For this review, take the finished solid that the model builds, in its own axes (mm). A direction names the side the tool comes from. Give positions to 0.01 mm unless a question says otherwise; leave off trailing zeros. Write each loop counter-clockwise with the first axis right and the second up, starting at its lowest first coordinate (ties: lowest second). Pieces come first, ordered by that corner, then holes.
1) We need section C-C on x = -27. Give the boundary of the cut face in (y, z), and give its area (3 significant figures).
2) Wall thickness on line 1 along Y through (x, z) = (0, 4); line 2 along Y through (x, z) = (-26.5, 0.75); line 3 along X through (y, z) = (8, 2.5): over which ranges is each line inside the solid? List them lowest first.
3) We need section D-D on x = -7.5. Give the boundary of the cut face in (y, z).
4) Machinability: for faces 5 (the face through (-22, 3.687, 3)), 6 (the face through (-29, 4.738, 3)), 7 (the face through (-31.567, -4, 3)), 8 (the face through (-0.22, -21.85, 7.49)), which of the approach directions +Z, -Z, +X, -X, +Y, -Y give a long, thin tool a straight path to every point of the face, cutting with its end or side? Answer none if there is none.
5) We need section B-B on x = 0. Give the boundary of the cut face in (y, z) (3 decimals), and give its area (3 significant figures).
6) For P1, Ø1.5, axis at x = 7, y = 14.5, coming from the +Z side; P2, Ø3.5, axis at x = -25.5, z = 3, coming from the +Y side, all flat-tipped, find the tip position at first contact; note any pin that passes through.
7) Draft analysis for pull direction Z (two halves, no side actions). For faces 1 (the face through (-27.028, -4.485, 1.426)), 2 (the face through (-28.3, -5.262, 1.9)), 3 (the face through (8, -10, 7)), 4 (the face through (-27.028, 4.205, 1.426)), state which applies: pulls with the +Z half, pulls with the -Z half, needs draft (parallel to the pull), parting line crosses it, or undercut.
8) We need section A-A on z = 3.5. Give the boundary of the cut face in (x, y), and give its area (3 significant figures).
from build123d import *

# Parameters (mm, degrees)
F1_DEPTH = 7
F2_R     = 2.125
F3_DEPTH = 10
F4_R     = 1
F5_DEPTH = 1


# Not quite as in the source:
# - a feature names something its author has since deleted; it is built from what else it names


with BuildPart() as f1:
    # F0 (on Top) → F1 (new body)
    with BuildSketch(Plane.XY):
        with BuildLine():
            ThreePointArc((-23.208916684, 3.6873006871), (-23.1191027664, 4.2139159074), (-23.017341427, 4.7383534726))
            Line((-23.017341427, 4.7383534726), (-31.5671088163, 4.7383534726))
            Line((-31.5671088163, 4.7383534726), (-31.5671088163, 3.6873006871))
            Line((-31.5671088163, 3.6873006871), (-23.208916684, 3.6873006871))
        make_face()
        with BuildLine():
            Line((-31.5671088163, -5.2616465274), (-22.9033856847, -5.2616465274))
            ThreePointArc((-22.9033856847, -5.2616465274), (-23.0695849256, -4.4770806738), (-23.208916684, -3.6873006871))
            Line((-23.208916684, -3.6873006871), (-31.5671088163, -3.6873006871))
            Line((-31.5671088163, -3.6873006871), (-31.5671088163, -5.2616465274))
        make_face()
        with BuildLine():
            ThreePointArc((-22.9033856847, -5.2616465274), (2.6476816661, -23.3503700569), (23.5, 0))
            ThreePointArc((23.5, 0), (2.3814361701, 23.3790239695), (-23.017341427, 4.7383534726))
            Line((-23.017341427, 4.7383534726), (-11.5671088163, 4.7383534726))
            ThreePointArc((-11.5671088163, 4.7383534726), (2.4146573045, 12.2645599229), (12.5, 0))
            ThreePointArc((12.5, 0), (2.4146573045, -12.2645599229), (-11.5671088163, -4.7383534726))
            Line((-11.5671088163, -4.7383534726), (-11.5671088163, -5.2616465274))
            Line((-11.5671088163, -5.2616465274), (-22.9033856847, -5.2616465274))
        make_face()
        with BuildLine():
            Line((-11.5671088163, 4.7383534726), (-23.017341427, 4.7383534726))
            ThreePointArc((-23.017341427, 4.7383534726), (-23.1191027664, 4.2139159074), (-23.208916684, 3.6873006871))
            Line((-23.208916684, 3.6873006871), (-11.9437771933, 3.6873006871))
            ThreePointArc((-11.9437771933, 3.6873006871), (-11.7671839549, 4.2170347131), (-11.5671088163, 4.7383534726))
        make_face()
        with BuildLine():
            ThreePointArc((-23.208916684, -3.6873006871), (-23.0695849256, -4.4770806738), (-22.9033856847, -5.2616465274))
            Line((-22.9033856847, -5.2616465274), (-11.5671088163, -5.2616465274))
            Line((-11.5671088163, -5.2616465274), (-11.5671088163, -4.7383534726))
            ThreePointArc((-11.5671088163, -4.7383534726), (-11.7671839549, -4.2170347131), (-11.9437771933, -3.6873006871))
            Line((-11.9437771933, -3.6873006871), (-23.208916684, -3.6873006871))
        make_face()
    extrude(amount=F1_DEPTH)

    # F2 (on face) → F3 (cut)
    with BuildSketch(Plane.XZ.offset(5.2616465274)):
        with Locations((-26.5671088163, 3.5)):
            Circle(F2_R)
    extrude(amount=-F3_DEPTH, mode=Mode.SUBTRACT)

    # F4 (on face) → F5 (join, symmetric)
    with BuildSketch(Plane.XY.offset(7)):
        with Locations((0, -20.875)):
            Circle(F4_R)
        with Locations((0, 20.875)):
            Circle(F4_R)
    extrude(amount=F5_DEPTH, both=True)


solid = f1.part
Results list:
1. outline: (-5.26, 0) - (-3.69, 0) - (-3.69, 1.42) - (-5.26, 1.42) - close; (-5.26, 5.58) - (-3.69, 5.58) - (-3.69, 7) - (-5.26, 7) - close; (3.69, 0) - (4.74, 0) - (4.74, 1.42) - (3.69, 1.42) - close; (3.69, 5.58) - (4.74, 5.58) - (4.74, 7) - (3.69, 7) - close
1. area: 7.45 mm2
2. line 1: y = -23.5 to -12.5, 12.5 to 23.5
2. line 2: y = -5.26 to -3.69, 3.69 to 4.74
2. line 3: x = -22.1 to -9.6, 9.6 to 22.1
3. outline: (-22.27, 0) - (-10, 0) - (-10, 7) - (-22.27, 7) - close; (10, 0) - (22.27, 0) - (22.27, 7) - (10, 7) - close
4. face 5: +Z, -Z, -X
4. face 6: +Z, -Z, -X, +Y
4. face 7: +Z, -Z, -X, +Y, -Y
4. face 8: +Z
5. outline: (-23.5, 0) - (-12.5, 0) - (-12.5, 7) - (-19.875, 7) - (-19.875, 8) - (-21.875, 8) - (-21.875, 7) - (-23.5, 7) - close; (12.5, 0) - (23.5, 0) - (23.5, 7) - (21.875, 7) - (21.875, 8) - (19.875, 8) - (19.875, 7) - (12.5, 7) - close
5. area: 158 mm2
6. P1: stops at z = 7
6. P2: stops at y = 4.74
7. face 1: undercut
7. face 2: needs draft
7. face 3: pulls with the +Z half
7. face 4: undercut
8. outline: (-31.57, -5.26) - (-28.69, -5.26) - (-28.69, -3.69) - (-31.57, -3.69) - close; (-31.57, 3.69) - (-28.69, 3.69) - (-28.69, 4.74) - (-31.57, 4.74) - close; (-24.44, -5.26) - (-22.9, -5.26) arc R23.5 ccw (long way) to (-23.02, 4.74) - (-24.44, 4.74) - (-24.44, 3.69) - (-11.94, 3.69) arc R12.5 cw (long way) to (-11.94, -3.69) - (-24.44, -3.69) - close
8. area: 1,170 mm2
